For this review, take the finished solid that the model builds, in its own axes (mm). Face numbers are marked on the shaded views. A direction names the side the tool comes from. Round coordinates to 2 decimals unless told otherwise and drop trailing zeros. Loops run counter-clockwise (first coordinate to the right, second up) from the corner with the lowest first, then second, coordinate; pieces in that order, holes last.
1. Consider section C-C on y = 28. State the section outline as (x, z) points, then the cut area to 3 significant figures.
2. Clearance check with flat-ended pins moving along their axes: pin 1 Ø6 at (x, y) = (34, 9) entering from +Z; pin 2 Ø3 at (x, y) = (-39.5, 21.5) entering from -Z; pin 3 Ø11 at (y, z) = (4.5, -31.5) entering from +X; pin 4 Ø18 at (x, z) = (0, 0) entering from -Y. State where each tip first meets the part, or that it passes through.
3. Tool access review of the marked faces 5, 6, 7, 8 and 9: name each direction out of +Z, -Z, +X, -X, +Y, -Y from which nothing blocks a thin tool from reaching the whole face with its end or side.
4. Draft analysis for pull direction Z (two halves, no side actions). For the marked faces 1, 2, 3 and 4, state which applies: released by +Z, released by -Z, zero draft, split by the parting line, or undercut.
5. To check wall thickness, follow line 1 along Z through (x, y) = (29, 7.5); line 2 along Z through (x, y) = (-43, 8.5); line 3 along Z through (x, y) = (5, 22). State the ranges of each line that lie inside material, in increasing order.
6. Consider section A-A on z = 0. State the section outline as (x, y) points.
7. Consider section B-B on x = 13.5. State the section outline as (y, z) points, then the cut area to 3 significant figures.
from build123d import *

# Parameters (mm, degrees)
SKETCH2_R           = 14.798837294
BOSS_EXTRUDE1_DEPTH = 10
SKETCH2_7_W         = 15
SKETCH2_7_H         = 11.547005384
BOSS_EXTRUDE3_DEPTH = 30
FILLET1_R           = 10


with BuildPart() as part:
    # Sketch2 → Boss-Extrude1 (new body)
    with BuildSketch(Plane(origin=(0, 0, 0), x_dir=(0, 0, -1), z_dir=(0, 1, 0))):
        with BuildLine():
            Line((-38.301270189, -11.339745962), (-43.301270189, -20))
            ThreePointArc((-43.301270189, -20), (-43.301270189, -25), (-38.97114317, -27.5))
            Line((-38.97114317, -27.5), (-28.97114317, -27.5))
            Line((-28.97114317, -27.5), (-13.97114317, -27.5))
            Line((-13.97114317, -27.5), (13.97114317, -27.5))
            Line((13.97114317, -27.5), (28.97114317, -27.5))
            Line((28.97114317, -27.5), (38.97114317, -27.5))
            ThreePointArc((38.97114317, -27.5), (43.301270189, -25), (43.301270189, -20))
            Line((43.301270189, -20), (38.301270189, -11.339745962))
            Line((38.301270189, -11.339745962), (30.801270189, 1.650635095))
            Line((30.801270189, 1.650635095), (16.830127019, 25.849364905))
            Line((16.830127019, 25.849364905), (9.330127019, 38.839745962))
            Line((9.330127019, 38.839745962), (4.330127019, 47.5))
            ThreePointArc((4.330127019, 47.5), (0, 50), (-4.330127019, 47.5))
            Line((-4.330127019, 47.5), (-9.330127019, 38.839745962))
            Line((-9.330127019, 38.839745962), (-16.830127019, 25.849364905))
            Line((-16.830127019, 25.849364905), (-30.801270189, 1.650635095))
            Line((-30.801270189, 1.650635095), (-38.301270189, -11.339745962))
        make_face()
        with Locations(Location((0, 0, 0), (0, 0, 180))):
            Circle(SKETCH2_R, mode=Mode.SUBTRACT)
    extrude(amount=BOSS_EXTRUDE1_DEPTH)

    # Sketch2_7 → Boss-Extrude3 (add)
    with BuildSketch(Plane(origin=(0, 0, 0), x_dir=(0, 0, -1), z_dir=(0, 1, 0))):
        Polygon((38.301270189, -11.339745962), (30.801270189, 1.650635095), (40.801270189, 7.424137787), (48.301270189, -5.56624327), align=None)
        with Locations((21.47114317, -33.273502692)):
            Rectangle(SKETCH2_7_W, SKETCH2_7_H)
        with Locations((-21.47114317, -33.273502692)):
            Rectangle(SKETCH2_7_W, SKETCH2_7_H)
        Polygon((-38.301270189, -11.339745962), (-48.301270189, -5.56624327), (-40.801270189, 7.424137787), (-30.801270189, 1.650635095), align=None)
        Polygon((-9.330127019, 38.839745962), (-16.830127019, 25.849364905), (-26.830127019, 31.622867597), (-19.330127019, 44.613248654), align=None)
        Polygon((9.330127019, 38.839745962), (19.330127019, 44.613248654), (26.830127019, 31.622867597), (16.830127019, 25.849364905), align=None)
    extrude(amount=BOSS_EXTRUDE3_DEPTH)

    # Fillet1
    fillet1_edges = [part.edges().sort_by_distance(p)[0] for p in [
        (-0.928947258, 0, -44.551270189),
        (-38.118058126, 0, -23.080127019),
        (-38.118058126, 0, 23.080127019),
        (-0.928947258, 0, 44.551270189),
        (39.047005384, 0, 21.47114317),
        (39.047005384, 0, -21.47114317),
    ]]
    fillet(fillet1_edges, radius=FILLET1_R)


solid = part.part
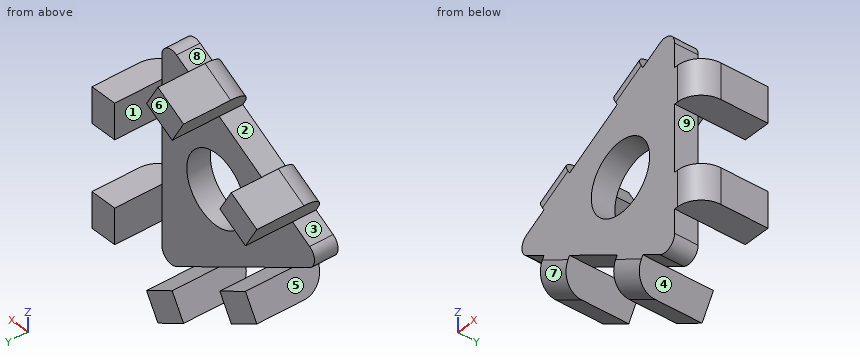
Resolved:
1. outline: (-44.61, -19.33) - (-31.62, -26.83) - (-25.85, -16.83) - (-38.84, -9.33) - close; (-44.61, 19.33) - (-38.84, 9.33) - (-25.85, 16.83) - (-31.62, 26.83) - close; (-7.42, -40.8) - (5.57, -48.3) - (11.34, -38.3) - (-1.65, -30.8) - close; (-7.42, 40.8) - (-1.65, 30.8) - (11.34, 38.3) - (5.57, 48.3) - close; (27.5, -28.97) - (39.05, -28.97) - (39.05, -13.97) - (27.5, -13.97) - close; (27.5, 13.97) - (39.05, 13.97) - (39.05, 28.97) - (27.5, 28.97) - close
1. area: 1,040 mm2
2. pin 1: stops at z = 28.97
2. pin 2: stops at z = -23.15
2. pin 3: stops at x = 39.03
2. pin 4: passes through
3. face 5: -X, +Y, -Y
3. face 6: +Z, -Z, +X, -X, +Y
3. face 7: -Z, -X, -Y
3. face 8: +Z, +Y, -Y
3. face 9: +X, +Y, -Y
4. face 1: zero draft
4. face 2: undercut
4. face 3: undercut
4. face 4: released by -Z
5. line 1: z = -28.97 to -13.97, 13.97 to 28.97
5. line 2: z = -20.13 to -16.54, -6.93 to 6.93, 16.54 to 20.13
5. line 3: z = -47.97 to -34.64, 34.64 to 47.97
6. outline: (-50, 0) - (-14.8, 0) - (-14.8, 10) - (-50, 10) - close; (14.8, 0) - (27.5, 0) - (27.5, 10) - (14.8, 10) - close
7. outline: (0, -39.55) - (10, -39.55) - (10, -6.06) - (0, -6.06) - close; (0, 6.06) - (10, 6.06) - (10, 39.55) - (0, 39.55) - close
7. area: 670 mm2
